Verification items for this drawing (mm, ordinates from the low corner). A direction names the side the tool comes from. Round coordinates to 2 decimals unless told otherwise and drop trailing zeros. Order: outer loops, then holes, each group sorted by start corner. A loop starts at its lowest first (then second) coordinate and runs counter-clockwise, first axis right, second up. Notation, with made-up numbers: (84, 38.5) -> (91, 38.5) arc R21 ccw to (91, 77.5) -> close; hole circle Ø2 at (69.5, 37.5). An arc over 180 degrees is marked (long way). Answer in a Markdown table with one row per item.
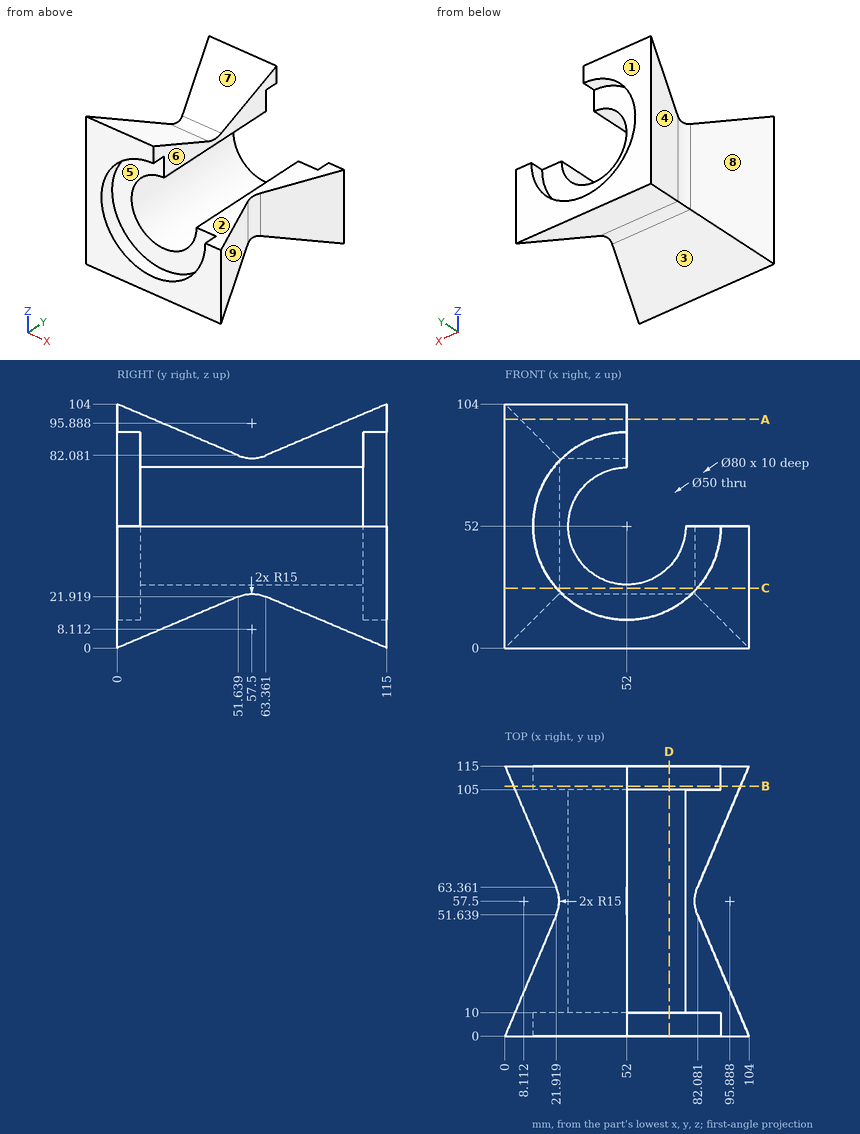
Item 1: Cross-section at C-C (z = 25.5). Record the boundary of the cut face in (x, y).
Result sheet:
| item | result |
|---|---|
| outline | (0, 0) -> (22.04, 0) -> (22.04, 10) -> (81.96, 10) -> (81.96, 0) -> (104, 0) -> (82.08, 51.64) arc R15 cw to (82.08, 63.36) -> (104, 115) -> (81.96, 115) -> (81.96, 105) -> (22.04, 105) -> (22.04, 115) -> (0, 115) -> (21.92, 63.36) arc R15 cw to (21.92, 51.64) -> close |
Item 2: Mould release check, pull along Y, two halves, no side actions. Record for the marked faces 1, 2, 3 and 4: pulls with the +Y half, pulls with the -Y half, needs draft (parallel to the pull), parting line crosses it, or undercut.
Result sheet:
| item | result |
|---|---|
| face 1 | pulls with the +Y half |
| face 2 | needs draft |
| face 3 | undercut |
| face 4 | undercut |
Item 3: Set-up check for the marked faces 5, 6, 7, 8 and 9: record each of +Z, -Z, +X, -X, +Y, -Y from which the full face is reachable in a straight line by a thin tool's end or side.
Result sheet:
| item | result |
|---|---|
| face 5 | -Y |
| face 6 | +Z, +X, +Y, -Y |
| face 7 | +Z, +X, -X |
| face 8 | +Z, -Z, -X |
| face 9 | +Z, -Z, +X |
Item 4: Cross-section at D-D (x = 70). Record the boundary of the cut face in (y, z), and give its area (3 significant figures).
Result sheet:
| item | result |
|---|---|
| outline | (0, 0) -> (51.64, 21.92) arc R15 cw to (63.36, 21.92) -> (115, 0) -> (115, 16.28) -> (105, 16.28) -> (105, 34.65) -> (10, 34.65) -> (10, 16.28) -> (0, 16.28) -> close |
| area | 2,220 mm^2 |
Item 5: Scan lines: line 1 (Y direction, x = 82, z = 12) (1 decimal); line 2 (Z direction, x = 32, y = 32) (1 decimal); line 3 (Y direction, x = 15.5, z = 55) (1 decimal). Record each from-to range of solid material in increasing order. Write a range as [from, to].
Result sheet:
| item | result |
|---|---|
| line 1 | y = [0, 28.3], [86.7, 115] |
| line 2 | z = [13.6, 37], [67, 90.4] |
| line 3 | y = [10, 36.5], [78.5, 105] |
Item 6: Depth check by flat-ended pin: P1, Ø1, axis at x = 53, y = 70.5, coming from the +Z side (1 decimal); P2, Ø8, axis at y = 90.5, z = 43.5, coming from the -X side; P3, Ø2, axis at x = 76.5, y = 84.5, coming from the -Z side. Enter the tip coordinate at first touch or a pass-through.
Result sheet:
| item | result |
|---|---|
| P1 | stops at z = 27 |
| P2 | stops at x = 8.7 |
| P3 | stops at z = 12.52 |
Item 7: Cross-section at B-B (y = 106.5). Record the boundary of the cut face in (x, z).
Result sheet:
| item | result |
|---|---|
| outline | (3.61, 3.61) -> (100.39, 3.61) -> (100.39, 52) -> (92, 52) arc R40 cw (long way) to (52, 92) -> (52, 100.39) -> (3.61, 100.39) -> close |
Item 8: Cross-section at A-A (z = 97.5). Record the boundary of the cut face in (x, y).
Result sheet:
| item | result |
|---|---|
| outline | (0, 0) -> (52, 0) -> (52, 15.31) -> (6.5, 15.31) -> close; (0, 115) -> (6.5, 99.69) -> (52, 99.69) -> (52, 115) -> close |
